Autodesk Inventor part; units mm, degrees
ref_plane "YZ Plane" through (0, 0, 0) normal (1, 0, 0) x (0, 1, 0)
ref_plane "XZ Plane" through (0, 0, 0) normal (0, 1, 0) x (-1, 0, 0)
ref_plane "XY Plane" through (0, 0, 0) normal (0, 0, 1) x (1, 0, 0)
sketch "Sketch2" plane through (0, 0, 0) normal (0, 0, 1) x (1, 0, 0)
  circle A0 centre (6, 6) radius 2
  circle A1 centre (0.0033, 31.0033) radius 1.6
  circle A2 centre (-31.0033, -0.0033) radius 1.6
  line L0 (-31.0033, -0.0033) -> (0.0033, 31.0033) construction
  arc A3 (-26.1066, 4.8934) -> (-4.8934, 26.1066) centre (-15.5, 15.5) ccw
  line L1 (-15.5, 15.5) -> (0, 0) construction
  arc A4 (0.0041, 37.9283) -> (-4.8934, 26.1066) centre (0.0033, 31.0033) ccw
  circle A5 centre (-6, -6) radius 2
  line L2 (6, 6) -> (-6, -6) construction
  arc A6 (26.8194, 26.8194) -> (0.0041, 37.9283) centre (0, 0) ccw
  line L3 (26.8194, 26.8194) -> (7.4142, 7.4142)
  arc A7 (-26.1066, 4.8934) -> (-37.9283, -0.0041) centre (-31.0033, -0.0033) ccw
  arc A8 (-37.9283, -0.0041) -> (-26.8194, -26.8194) centre (0, 0) ccw
  line L4 (-26.8194, -26.8194) -> (-7.4142, -7.4142)
  line L5 (-4.5858, -4.5858) -> (4.5858, 4.5858)
  dimension "d0" = 6
  dimension "d1" = 6
  dimension "d2" = 4
  dimension "d3" = 43.85
  dimension "d4" = 3.2
  dimension "d5" = 30
  dimension "d6" = 15.5
  dimension "d7" = 15.5
extrude "Extrusion1" add sketch "Sketch2" along normal blind 2.5 contours A0 L5 A5 L4 A8 A7 A3 A4 A6 L3
mirror "Mirror1" about plane through (-4.5858, -4.5858, 0) normal (0.7071, -0.7071, 0)
equation "\"d1\" = d0"
equation "\"d7\" = d6"
properties part number "mount-plate_3DPrint"
The listing builds one solid part. Answer for the finished solid, in the listing's coordinates (mm). Coordinates: 2 decimals unless noted, no trailing zeros. Loops run counter-clockwise (first coordinate to the right, second up) from the corner with the lowest first, then second, coordinate; pieces in that order, holes last.
1) Flat-ended cylindrical pins translate along their axes: pin 1 Ø1.5 at (x, z) = (-16, 1) entering from -Y; pin 2 Ø3 at (x, y) = (6, 6) entering from -Z. Find the tip coordinate at first contact, or state that the pin passes through.
2) Find section D-D on y = 15.5. Write down the section's boundary in (x, z).
3) Determine the mould class of faces 1 (the face through (6.437, -33.548, 1.232)), 2 (the face through (-0.344, 32.565, 1.232)), 3 (the face through (-1, 1, 0)) for opening direction Y: pulls with the +Y half, pulls with the -Y half, needs draft (parallel to the pull), parting line crosses it, or undercut.
4) Find section B-B on x = 6. Write down the section's boundary in (y, z), then the cut area to 3 significant figures.
5) Find section A-A on y = -6. Write down the section's boundary in (x, z).
6) Find section C-C on z = 1.15. Write down the section's boundary in (x, y) (3 decimals), then the cut area to 3 significant figures.
7) Find the intervals of material crossed by L1, parallel to Y at x = -6, z = 1.35; L2, parallel to Y at x = -2, z = 0.6, in increasing order.
Values:
1. pin 1: stops at y = -34.73
1. pin 2: passes through
2. outline: (-0.5, 0) - (34.62, 0) - (34.62, 2.5) - (-0.5, 2.5) - close
3. face 1: undercut
3. face 2: undercut
3. face 3: needs draft
4. outline: (-34.46, 0) - (-27.55, 0) - (-27.55, 2.5) - (-34.46, 2.5) - close; (-3.89, 0) - (4, 0) - (4, 2.5) - (-3.89, 2.5) - close; (8, 0) - (37.45, 0) - (37.45, 2.5) - (8, 2.5) - close
4. area: 111 mm2
5. outline: (-37.45, 0) - (-8, 0) - (-8, 2.5) - (-37.45, 2.5) - close; (-4, 0) - (3.89, 0) - (3.89, 2.5) - (-4, 2.5) - close; (27.55, 0) - (34.46, 0) - (34.46, 2.5) - (27.55, 2.5) - close
6. outline: (-37.928, -0.004) arc R37.929 ccw to (-26.819, -26.819) arc R37.929 ccw to (-0.004, -37.928) arc R6.925 ccw to (4.893, -26.107) arc R15 cw to (26.107, -4.893) arc R6.925 ccw to (37.928, 0.004) arc R37.928 ccw to (26.819, 26.819) arc R37.928 ccw to (0.004, 37.928) arc R6.925 ccw to (-4.893, 26.107) arc R15 cw to (-26.107, 4.893) arc R6.925 ccw to start; hole circle Ø3.2 at (-31.003, -0.003); hole circle Ø4 at (-6, -6); hole circle Ø3.2 at (-0.003, -31.003); hole circle Ø3.2 at (0.003, 31.003); hole circle Ø4 at (6, 6); hole circle Ø3.2 at (31.003, 0.003)
6. area: 2,680 mm2
7. L1: y = -37.45 to -8, -4 to 3.89, 27.55 to 34.46
7. L2: y = -37.88 to 8.96, 22.04 to 37.63
